```python
from build123d import *

# Parameters (mm, degrees)
SKETCH1_W           = 5
SKETCH1_H           = 25
SKETCH1_H_2         = 20
BOSS_EXTRUDE2_DEPTH = 5


with BuildPart() as part:
    # Sketch1 → Boss-Extrude2 (new body)
    with BuildSketch(Plane(origin=(0, 0, 0), x_dir=(1, 0, 0), z_dir=(0, 1, 0))):
        Polygon((-24.829979235, 345.545008259), (-19.829979235, 345.545008259), (-19.829979235, 335.545008259), (-24.829979235, 335.545008259), (-24.829979235, 325.545008259), (-19.829979235, 325.545008259), (-19.829979235, 315.545008259), (-19.829979235, 305.545008259), (-24.829979235, 305.545008259), (-24.829979235, 295.545008259), (-19.829979235, 295.545008259), (-19.829979235, 285.545008259), (-19.829979235, 275.545008259), (-24.829979235, 275.545008259), (-24.829979235, 265.545008259), (-19.829979235, 265.545008259), (-19.829979235, 255.545008259), (-19.829979235, 245.545008259), (-24.829979235, 245.545008259), (-24.829979235, 235.545008259), (-19.829979235, 235.545008259), (-19.829979235, 225.545008259), (-19.829979235, 215.545008259), (-24.829979235, 215.545008259), (-24.829979235, 205.545008259), (-19.829979235, 205.545008259), (-19.829979235, 195.545008259), (-19.829979235, 185.545008259), (-24.829979235, 185.545008259), (-24.829979235, 175.545008259), (-19.829979235, 175.545008259), (-19.829979235, 165.545008259), (-19.829979235, 155.545008259), (-24.829979235, 155.545008259), (-24.829979235, 145.545008259), (-19.829979235, 145.545008259), (-19.829979235, 135.545008259), (-19.829979235, 125.545008259), (-24.829979235, 125.545008259), (-24.829979235, 115.545008259), (-19.829979235, 115.545008259), (-19.829979235, 105.545008259), (-19.829979235, 95.545008259), (-24.829979235, 95.545008259), (-24.829979235, 85.545008259), (-19.829979235, 85.545008259), (-19.829979235, 75.545008259), (-19.829979235, 65.545008259), (-24.829979235, 65.545008259), (-24.829979235, 55.545008259), (-19.829979235, 55.545008259), (-19.829979235, 45.545008259), (-19.829979235, 35.545008259), (-24.829979235, 35.545008259), (-24.829979235, 25.545008259), (-19.829979235, 25.545008259), (-19.829979235, 15.545008259), (-25.820121993, 15.545008259), (-25.676959723, 5.546033083), (276.017001253, 5.546033083), (276.160163523, 15.545008259), (270.170020765, 15.545008259), (270.170020765, 25.545008259), (275.170020765, 25.545008259), (275.170020765, 35.545008259), (270.170020765, 35.545008259), (270.170020765, 45.545008259), (270.170020765, 55.545008259), (275.170020765, 55.545008259), (275.170020765, 65.545008259), (270.170020765, 65.545008259), (270.170020765, 75.545008259), (270.170020765, 85.545008259), (275.170020765, 85.545008259), (275.170020765, 95.545008259), (270.170020765, 95.545008259), (270.170020765, 105.545008259), (270.170020765, 115.545008259), (275.170020765, 115.545008259), (275.170020765, 125.545008259), (270.170020765, 125.545008259), (270.170020765, 135.545008259), (270.170020765, 145.545008259), (275.170020765, 145.545008259), (275.170020765, 155.545008259), (270.170020765, 155.545008259), (270.170020765, 165.545008259), (270.170020765, 175.545008259), (275.170020765, 175.545008259), (275.170020765, 185.545008259), (270.170020765, 185.545008259), (270.170020765, 195.545008259), (270.170020765, 205.545008259), (275.170020765, 205.545008259), (275.170020765, 215.545008259), (270.170020765, 215.545008259), (270.170020765, 225.545008259), (270.170020765, 235.545008259), (275.170020765, 235.545008259), (275.170020765, 245.545008259), (270.170020765, 245.545008259), (270.170020765, 255.545008259), (270.170020765, 265.545008259), (275.170020765, 265.545008259), (275.170020765, 275.545008259), (270.170020765, 275.545008259), (270.170020765, 285.545008259), (270.170020765, 295.545008259), (275.170020765, 295.545008259), (275.170020765, 305.545008259), (270.170020765, 305.545008259), (270.170020765, 315.545008259), (270.170020765, 325.545008259), (275.170020765, 325.545008259), (275.170020765, 335.545008259), (270.170020765, 335.545008259), (270.170020765, 345.545008259), (275.170020765, 345.545008259), (275.170020765, 355.545008259), (-24.829979235, 355.545008259), align=None)
        with Locations((125.170020765, 313.045008259)):
            Rectangle(SKETCH1_W, SKETCH1_H, mode=Mode.SUBTRACT)
        with Locations((125.170020765, 48.046033083)):
            Rectangle(SKETCH1_W, SKETCH1_H, mode=Mode.SUBTRACT)
        with Locations((125.170020765, 250.545008259)):
            Rectangle(SKETCH1_W, SKETCH1_H_2, mode=Mode.SUBTRACT)
        with Locations((125.170020765, 110.546033083)):
            Rectangle(SKETCH1_W, SKETCH1_H_2, mode=Mode.SUBTRACT)
    extrude(amount=BOSS_EXTRUDE2_DEPTH)


solid = part.part
```
For this review, take the finished solid that the model builds, in its own axes (mm). Give positions to 0.01 mm unless a question says otherwise; leave off trailing zeros. Write each loop counter-clockwise with the first axis right and the second up, starting at its lowest first coordinate (ties: lowest second). Pieces come first, ordered by that corner, then holes. Notation, with made-up numbers: M 33,12.25 L 92,12.25 A20 ccw 92,41.25 Z; hole C 60,-18 d10. An arc over 180 degrees is marked long. Answer as a JSON object with one key per item and string values. Group by question number.
Item 1: Consider section B-B on z = -191. Write out the cut boundary in (x, y), plus the area to 3 significant figures.
Item 2: Consider section A-A on z = -315. Write out the cut boundary in (x, y), plus the area to 4 significant figures.
Item 3: For probe 1 along X at (y, z) = (2.4, -109.5); probe 2 along X at (y, z) = (1.95, -213.5); probe 3 along X at (y, z) = (2.7, -294), list the stretches that pass through material, from the lowest coordinate up. Write a range as [from, to].
Item 4: For pin 1 Ø2.5 at (y, z) = (1.5, -316) entering from -X; pin 2 Ø2.5 at (y, z) = (2, -115.5) entering from +X; pin 3 Ø2.5 at (y, z) = (3.5, -329.5) entering from -X, all flat-tipped, find the tip position at first contact; note any pin that passes through.
Check result:
{
 "1": {"outline": "M -19.83,0 L 270.17,0 L 270.17,5 L -19.83,5 Z", "area": "1,450 mm^2"},
 "2": {"outline": "M -19.83,0 L 122.67,0 L 122.67,5 L -19.83,5 Z; M 127.67,0 L 270.17,0 L 270.17,5 L 127.67,5 Z", "area": "1,425 mm^2"},
 "3": {"probe 1": "x = [-19.83, 122.67], [127.67, 270.17]", "probe 2": "x = [-24.83, 275.17]", "probe 3": "x = [-19.83, 270.17]"},
 "4": {"pin 1": "stops at x = -19.83", "pin 2": "stops at x = 275.17", "pin 3": "stops at x = -24.83"}
}
